Read the model definition and answer for the solid it produces. Units are mm, in the model's axes. Face numbers are marked on the shaded views. A direction names the side the tool comes from. Coordinates: 2 decimals unless noted, no trailing zeros. Loops run counter-clockwise (first coordinate to the right, second up) from the corner with the lowest first, then second, coordinate; pieces in that order, holes last. Notation, with made-up numbers: (77.25, 8) -> (120.25, 8) arc R10 cw to (120.25, 27) -> close; hole circle Ø5 at (10, 12). An arc over 180 degrees is marked (long way). Answer as a JSON object with one key per item and string values. Group by question number.
Q1. The part is cut by section C-C on x = -81.75. Write down the section's boundary in (y, z).
Q2. The part is cut by section D-D on y = 4. Write down the section's boundary in (x, z).
Q3. Each of these flat-tipped pins is pushed along its axis until it touches: P1, Ø3, axis at x = -10, z = -10, coming from the -Y side; P2, Ø5, axis at y = 5.5, z = -11, coming from the +X side; P3, Ø1, axis at y = 11.5, z = -52, coming from the -X side; P4, Ø5, axis at x = -84.5, y = 13.5, coming from the -Z side. Where does it stop, or does it pass through?
Q4. Straight lines are drawn through the part: line 1 along Z through (x, y) = (-88.25, 3); line 2 along Z through (x, y) = (-10, 13.75); line 3 along X through (y, z) = (7.5, -51.75). For each, find the intervals that lie inside material, in ascending order. Write a range as [from, to].
Q5. The part is cut by section B-B on z = -10. Write down the section's boundary in (x, y).
Q6. The part is cut by section A-A on x = -10. Write down the section's boundary in (y, z).
Q7. For the marked faces 1, 2 and 3, determine the directions among +Z, -Z, +X, -X, +Y, -Y from which every point of the face is accessible in a straight line to the end or side of a thin tool.
Autodesk Inventor part; units mm, degrees
ref_plane "YZ Plane" through (0, 0, 0) normal (1, 0, 0) x (0, 1, 0)
ref_plane "XZ Plane" through (0, 0, 0) normal (0, 1, 0) x (-1, 0, 0)
ref_plane "XY Plane" through (0, 0, 0) normal (0, 0, 1) x (1, 0, 0)
sketch "Boceto1" plane through (0, 0, 0) normal (0, 1, 0) x (-1, 0, 0)
  line L0 (100, 80) -> (-100, 80)
  line L1 (-100, 80) -> (-100, -80)
  line L2 (-100, -80) -> (100, -80)
  line L3 (100, -80) -> (100, 80)
  line L4 (100, 80) -> (-100, -80) construction
  line L5 (-100, 80) -> (100, -80) construction
  point P0 (0, 0)
  dimension "d0" = 200
  dimension "d1" = 160
extrude "Extrusión1" add sketch "Boceto1" along normal blind 20
sketch "Boceto2" plane through (0, 20, 0) normal (0, 1, 0) x (1, 0, 0)
  line L0 (-100, 80) -> (-100, -80)
  line L1 (-100, 80) -> (-70, 80)
  line L2 (-70, 80) -> (-70, 40)
  line L3 (-70, 40) -> (-100, 40)
  line L4 (-100, 40) -> (-100, 80)
  line L5 (100, 80) -> (-100, 80)
  line L6 (0, 80) -> (0, 40)
  line L7 (100, 80) -> (70, 80)
  line L8 (70, 80) -> (70, 40)
  line L9 (70, 40) -> (100, 40)
  line L10 (100, 40) -> (100, 80)
  point P0 (0, 0)
  dimension "d4" = 30
  dimension "d5" = 40
extrude "Extrusión2" cut sketch "Boceto2" against normal blind 10
sketch "Boceto3" plane through (0, 20, 0) normal (0, 1, 0) x (1, 0, 0)
  line L0 (-70, 80) -> (-70, 40)
  line L1 (-70, 80.0001) -> (-70, 40)
  line L2 (-70, 40) -> (-100, 40)
  line L3 (-100, 40) -> (-100, 80.0001)
  line L4 (-100, 40) -> (-70, 40)
  line L5 (-70, 40) -> (-70, 80)
  line L6 (-70, 80) -> (-100, 80)
  line L7 (-100, 80) -> (-100, 40)
  circle A0 centre (-88.25, 58.25) radius 1.75
  circle A1 centre (-81.75, 51.75) radius 1.75
  line L8 (100, 80) -> (-100, 80)
  line L9 (0, 80) -> (0, 56.5)
  circle A2 centre (88.25, 58.25) radius 1.75
  circle A3 centre (81.75, 51.75) radius 1.75
  point P0 (0, 0)
  point P1 (-64.3507, 80)
  point P2 (-74.3507, 0)
  point P3 (-85, 80)
  dimension "d23" = 21.75
  dimension "d24" = 11.75
  dimension "d26" = 11.75
hole "Agujero1" at (-81.75, 20, -51.75) at (-88.25, 20, -58.25) at (81.75, 20, -51.75) at (88.25, 20, -58.25) direction (0, -1, 0) diameter 3.5 end through all
sketch "Boceto4" plane through (-100, 0, 80) normal (0, 0, 1) x (1, 0, 0)
  line L0 (30, 20) -> (60, 20)
  line L1 (60, 20) -> (60, 10)
  line L2 (60, 10) -> (30, 10)
  line L3 (30, 10) -> (30, 20)
  line L4 (0, 0) -> (0, 20)
  line L5 (100, 0) -> (100, 10)
  line L6 (170, 20) -> (140, 20)
  line L7 (140, 20) -> (140, 10)
  line L8 (140, 10) -> (170, 10)
  line L9 (170, 10) -> (170, 20)
  dimension "d34" = 30
  dimension "d35" = 10
  dimension "d36" = 30
extrude "Extrusión3" add sketch "Boceto4" along normal blind 40
sketch "Boceto5" plane through (0, 20, 0) normal (0, 1, 0) x (1, 0, 0)
  line L0 (59.9999, -50) -> (69.9999, -50)
  line L1 (49.9999, -101.75) -> (49.9999, -79.9497)
  line L2 (59.9999, -108.25) -> (59.9999, -50)
  line L3 (40, -80) -> (69.9999, -80)
  line L4 (49.9999, -79.9497) -> (40, -80)
  circle A0 centre (51.7499, -101.75) radius 1.75
  circle A1 centre (58.2499, -108.25) radius 1.75
  line L5 (69.9999, -80) -> (69.9999, -120)
  line L6 (40, -120) -> (40, -80)
  line L7 (69.9999, -120) -> (40, -120)
  line L8 (0, -50) -> (0, -71.75)
  line L9 (-40, -120) -> (-40, -80)
  line L10 (-49.9999, -101.75) -> (-49.9999, -79.9497)
  circle A2 centre (-51.7499, -101.75) radius 1.75
  circle A3 centre (-58.2499, -108.25) radius 1.75
  line L11 (-40, -80) -> (-69.9999, -80)
  line L12 (-69.9999, -120) -> (-40, -120)
  line L13 (-69.9999, -80) -> (-69.9999, -120)
  line L14 (-59.9999, -108.25) -> (-59.9999, -50)
  line L15 (-40, -120) -> (-69.9999, -120)
  line L16 (-69.9999, -80) -> (-69.9999, -120)
  line L17 (-40, -120) -> (-70, -120)
  line L18 (-40, -80) -> (-40, -120)
  line L19 (-59.9999, -110) -> (-49.9999, -110)
  line L20 (-49.9999, -110) -> (-49.9999, -100)
  line L21 (-49.9999, -100) -> (-59.9999, -100)
  line L22 (-59.9999, -100) -> (-59.9999, -110)
  line L23 (-100, 40) -> (-100, -80)
  point P0 (0, 0)
  point P1 (-56.75, -68.25)
  point P2 (-63.25, -61.75)
  point P3 (63.25, -61.75)
  point P4 (56.75, -68.25)
  dimension "d45" = 3.5
  dimension "d46" = 3.5
  dimension "d39" = 10
  dimension "d40" = 10
  dimension "d41" = 40
  dimension "d42" = 0
  dimension "d43" = 6.5
  dimension "d44" = 6.5
  dimension "d47" = 11.7499
  dimension "d48" = 11.75
  dimension "d49" = 0
  dimension "d50" = 11.75
  dimension "d51" = 0
  dimension "d97" = 40.0001
hole "Agujero2" at (-58.2499, 20, 108.25) at (-51.7499, 20, 101.75) at (51.7499, 20, 101.75) at (58.2499, 20, 108.25) direction (0, -1, 0) diameter 3.5 end through all
sketch "Boceto6" plane through (0, 20, 0) normal (0, 1, 0) x (1, 0, 0)
  circle A0 centre (-60.569, -13.1067) radius 10
  circle A1 centre (-29.569, -59.1067) radius 3.5
  line L0 (-60.569, -13.1067) -> (-39.0083, -13.1067)
  circle A2 centre (-29.569, 25.8933) radius 3.5
  circle A3 centre (-88.569, 25.8933) radius 3.5
  circle A4 centre (-88.569, -59.1067) radius 3.5
  line L1 (70.4544, -63.0517) -> (18.4544, -63.0517)
  line L2 (18.4544, -63.0517) -> (18.4544, 6.9483)
  line L3 (18.4544, 6.9483) -> (70.4544, 6.9483)
  line L4 (70.4544, 6.9483) -> (70.4544, -63.0517)
  line L5 (70.4544, 6.9483) -> (48.4544, 6.9483)
  line L6 (48.4544, 6.9483) -> (48.4544, 48.9483)
  line L7 (48.4544, 48.9483) -> (70.4544, 48.9483)
  line L8 (70.4544, 48.9483) -> (70.4544, 6.9483)
  line L9 (77.2288, -8.158) -> (77.2281, -5.6604)
  circle A5 centre (63.7706, -5.7606) radius 1.75
  line L10 (70.7641, -24.1464) -> (70.7641, 22.2796)
  circle A6 centre (35.8307, -5.7609) radius 1.75
  line L11 (25.1581, -13.2381) -> (25.1581, -10.7404)
  circle A7 centre (68.8507, -57.8309) radius 1.75
  line L12 (26.4277, 35.0051) -> (26.4277, 37.5029)
  circle A8 centre (20.6074, -56.5614) radius 1.75
  line L13 (18.6941, -55.9176) -> (70.7641, -55.9176)
  line L14 (18.6941, -55.9176) -> (18.6941, -7.6743)
  line L15 (44.7291, -55.9176) -> (44.7291, -31.7959)
  line L16 (63.7706, -28.0517) -> (26.4277, -28.0517)
  line L17 (44.7291, -23.5247) -> (44.7291, -31.7959)
  point P0 (0, 0)
  point P1 (-60.569, -16.6067)
  point P2 (45.425, 12.8886)
  point P3 (44.7291, -28.0517)
  dimension "d59" = 7
  dimension "d60" = 7
  dimension "d61" = 7
  dimension "d62" = 39
  dimension "d63" = 46
  dimension "d64" = 59
  dimension "d65" = 46
  dimension "d66" = 39
  dimension "d67" = 59
  dimension "d68" = 52
  dimension "d69" = 70
  dimension "d70" = 22
  dimension "d71" = 42
  dimension "d72" = 3.5
  dimension "d73" = 3.5
  dimension "d74" = 3.5
  dimension "d75" = 3.5
  dimension "d142" = 17.3763
  dimension "d143" = 12.7092
  dimension "d144" = 6.6837
  dimension "d145" = 12.7089
  dimension "d146" = 5.2208
  dimension "d147" = 1.6037
  dimension "d148" = 2.1531
  dimension "d149" = 6.4903
hole "Agujero3" at (68.8507, 20, 57.8309) at (20.6074, 20, 56.5614) at (63.7706, 20, 5.7606) at (35.8307, 20, 5.7609) direction (0, -1, 0) diameter 3.5 end through all
sketch "Boceto7" plane through (0, 20, 0) normal (0, 1, 0) x (1, 0, 0)
  circle A0 centre (-60.569, -13.1067) radius 10
  circle A1 centre (-29.569, -59.1067) radius 3.5
  line L0 (-60.569, -13.1067) -> (-39.0083, -13.1067)
  circle A2 centre (-29.569, 25.8933) radius 3.5
  circle A3 centre (-88.569, 25.8933) radius 3.5
  circle A4 centre (-88.569, -59.1067) radius 3.5
  point P0 (0, 0)
  point P1 (-60.569, -16.6067)
  dimension "d83" = 7
  dimension "d84" = 7
  dimension "d85" = 7
  dimension "d86" = 39
  dimension "d87" = 46
  dimension "d88" = 59
  dimension "d89" = 46
  dimension "d90" = 39
  dimension "d91" = 59
extrude "Extrusión4" cut sketch "Boceto7" against normal blind 20
ref_plane "Plano de trabajo1" through (0, 0, -80) normal (-1, 0, 0) x (0, 0, 1)
ref_plane "Plano de trabajo2" through (100, 0, 0) normal (0, 0, -1) x (-1, 0, 0)
sketch "Boceto8" plane through (0, 20, 0) normal (0, 1, 0) x (1, 0, 0)
  line L0 (80, -15) -> (90, -15)
  circle A0 centre (85, -10) radius 1.75
  line L1 (85, 10) -> (85, -10)
  line L2 (90, -15) -> (90, 15)
  circle A1 centre (85, 10) radius 1.75
  line L3 (80, 15) -> (80, -15)
  line L4 (90, 15) -> (80, -15) construction
  line L5 (80, 15) -> (90, -15) construction
  line L6 (90, 15) -> (80, 15)
  line L7 (100, -80) -> (100, 40)
  line L8 (0, 0) -> (20, -20)
  line L9 (0, 0) -> (28.2843, 0) construction
  line L10 (15, -60) -> (15, -70)
  circle A2 centre (10, -65) radius 1.75
  line L11 (-10, -65) -> (10, -65)
  line L12 (15, -70) -> (-15, -70)
  circle A3 centre (-10, -65) radius 1.75
  line L13 (-15, -60) -> (15, -60)
  line L14 (-15, -70) -> (15, -60) construction
  line L15 (-15, -60) -> (15, -70) construction
  line L16 (-15, -70) -> (-15, -60)
  line L17 (0, 0) -> (18.6615, 18.6615)
  line L18 (0, 0) -> (26.3913, 0) construction
  line L19 (-15, 60) -> (-15, 70)
  circle A4 centre (-10, 65) radius 1.75
  line L20 (10, 65) -> (-10, 65)
  line L21 (-15, 70) -> (15, 70)
  circle A5 centre (10, 65) radius 1.75
  line L22 (15, 60) -> (-15, 60)
  line L23 (15, 70) -> (-15, 60) construction
  line L24 (15, 60) -> (-15, 70) construction
  line L25 (15, 70) -> (15, 60)
  line L26 (70, 80) -> (-70, 80)
  line L27 (-40, -80) -> (40, -80)
  point P0 (86.9608, 0)
  point P1 (86.9608, 0)
  point P2 (85, 15)
  point P3 (0, -69.1269)
  point P4 (0, -69.1269)
  point P5 (-15, -67.1661)
  point P6 (0, 69.7066)
  point P7 (0, 69.7066)
  point P8 (15, 67.7458)
  point P9 (-15, 65)
  point P10 (15, -65)
  dimension "d98" = 10
  dimension "d99" = 30
  dimension "d100" = 10
  dimension "d101" = 5
  dimension "d102" = 5
  dimension "d103" = 5
  dimension "d104" = 5
  dimension "d105" = 45
  dimension "d106" = 45
  dimension "d107" = 10
  dimension "d108" = 10
  dimension "d109" = 30
  dimension "d110" = 5
  dimension "d111" = 5
  dimension "d112" = 5
  dimension "d113" = 5
  dimension "d114" = 10
  dimension "d115" = 30
  dimension "d116" = 5
  dimension "d117" = 5
  dimension "d118" = 5
  dimension "d119" = 5
  dimension "d120" = 10
hole "Agujero4" at (-10, 20, -65) at (10, 20, -65) at (85, 20, -10) at (85, 20, 10) at (10, 20, 65) at (-10, 20, 65) direction (0, -1, 0) diameter 3.5 end through all
sketch "Boceto9" plane through (0, 20, 0) normal (0, 1, 0) x (1, 0, 0)
  circle A0 centre (10, -10) radius 1.75
  line L0 (6.803, 0) -> (14.6069, 0)
  line L1 (0, 0) -> (0, -4.8284)
  line L2 (0, 0) -> (20.0354, 0)
  circle A1 centre (10, 10) radius 1.75
  line L3 (0, 0) -> (0, 4.8284)
  circle A2 centre (-10, 10) radius 1.75
  circle A3 centre (-10, -10) radius 1.75
  dimension "d128" = 3.5
  dimension "d129" = 10
  dimension "d130" = 10
hole "Agujero5" at (-10, 20, 10) at (-10, 20, -10) at (10, 20, -10) at (10, 20, 10) direction (0, -1, 0) diameter 3.5 end through all
sketch "Boceto10" plane through (0, 0, 0) normal (0, -1, 0) x (1, 0, 0)
  line L0 (-16, 16) -> (16, 16)
  line L1 (16, 16) -> (16, -16)
  line L2 (16, -16) -> (-16, -16)
  line L3 (-16, -16) -> (-16, 16)
  line L4 (-16, 16) -> (16, -16) construction
  line L5 (16, 16) -> (-16, -16) construction
  point P0 (0, 0)
  point P1 (0, 0)
  dimension "d138" = 32
  dimension "d139" = 32
extrude "Extrusión5" cut sketch "Boceto10" against normal blind 10
split "Dividir1" plane through (100, 0, 0) removes the side toward (0, 0, 1)
split "Dividir2" plane through (0, 0, -80) removes the side toward (1, 0, 0)
properties part number "base_mid_1"
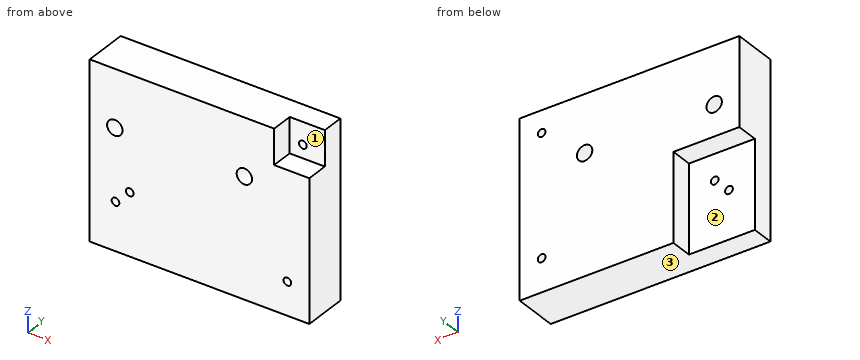
Final values:
{
 "1": {"outline": "(0, -80) -> (10, -80) -> (10, -53.5) -> (0, -53.5) -> close; (0, -50) -> (10, -50) -> (10, -40) -> (20, -40) -> (20, 0) -> (0, 0) -> close"},
 "2": {"outline": "(-100, -80) -> (0, -80) -> (0, -16) -> (-16, -16) -> (-16, 0) -> (-100, 0) -> close; hole circle Ø7 at (-88.57, -25.89); hole circle Ø3.5 at (-88.25, -58.25); hole circle Ø3.5 at (-81.75, -51.75); hole circle Ø7 at (-29.57, -25.89); hole circle Ø3.5 at (-10, -65)"},
 "3": {"P1": "passes through", "P2": "stops at x = -16", "P3": "stops at x = -70", "P4": "stops at z = -40"},
 "4": {"line 1": "z = [-80, -60], [-56.5, -29.38], [-22.41, 0]", "line 2": "z = [-80, -66.75], [-63.25, -11.75], [-8.25, 0]", "line 3": "x = [-100, -83.5], [-80, 0]"},
 "5": {"outline": "(-100, 0) -> (-16, 0) -> (-16, 10) -> (-11.75, 10) -> (-11.75, 20) -> (-100, 20) -> close; (-8.25, 10) -> (0, 10) -> (0, 20) -> (-8.25, 20) -> close"},
 "6": {"outline": "(0, -80) -> (20, -80) -> (20, -66.75) -> (0, -66.75) -> close; (0, -63.25) -> (20, -63.25) -> (20, -11.75) -> (10, -11.75) -> (10, -16) -> (0, -16) -> close; (10, -8.25) -> (20, -8.25) -> (20, 0) -> (10, 0) -> close"},
 "7": {"face 1": "+Z, +X, -Y", "face 2": "-Z, -X, +Y", "face 3": "-Z, +X, -X, +Y, -Y"}
}
